Read the model definition and answer for the solid it produces. Units are mm, in the model's axes. Face numbers are marked on the shaded views. A direction names the side the tool comes from. Give positions to 0.01 mm unless a question says otherwise; leave off trailing zeros. Write each loop counter-clockwise with the first axis right and the second up, starting at its lowest first coordinate (ties: lowest second). Pieces come first, ordered by that corner, then holes. Notation, with made-up numbers: (11, -7.5) -> (52, -7.5) arc R18 cw to (52, -3.5) -> close; hole circle Ø3 at (-23, 35). An arc over 180 degrees is marked (long way). Answer as CSV lines item,"result". Start each with the question number.
1. The part is cut by section A-A, the plane z = -3.25. Determine the outline of the cut face in (x, y), and give its area (3 significant figures).
2. The part is cut by section D-D, the plane z = 0. Determine the outline of the cut face in (x, y), and give its area (3 significant figures).
3. The part is cut by section C-C, the plane y = 1.5. Determine the outline of the cut face in (x, z).
4. Find the intervals of material crossed by line 1 (Z direction, x = 0, y = 5); line 2 (Z direction, x = 13, y = -42.5); line 3 (Y direction, x = -19, z = -1.5), in increasing order.
5. A tool of negligible diameter and unlimited length cuts with its end or side. For the marked faces 1, 2, 3, 4 and 5, from which of +Z, -Z, +X, -X, +Y, -Y can it reach the whole face along a straight path? Write none if from no direction.
6. The part is cut by section B-B, the plane x = 0. Determine the outline of the cut face in (y, z), and give its area (3 significant figures).
7. Given pin 1 (1 mm diameter, centred on y = -4, z = 3, fed in from -X); pin 2 (4 mm diameter, centred on x = -6.5, z = 2, fed in from +Y); pin 3 (3 mm diameter, centred on y = -22.5, z = 3.5, fed in from +X), each flat-ended and moving along its own axis, determine where each tip first touches the part or whether it passes through.
8. For a pull along X with two mould halves and no side action, classify the marked faces 6, 7 and 8 as pulls with the +X half, pulls with the -X half, needs draft (parallel to the pull), parting line crosses it, or undercut.
from build123d import *

# Parameters (mm, degrees)
PAD_DEPTH            = 4.5
SKETCH001_R          = 1
POCKET_DEPTH         = 11.302669
POCKET001_DEPTH      = 38.049191
POCKET001_DEPTH_BACK = -38.049191
FILLET_R             = 10


with BuildPart() as part:
    # Sketch → Pad (new body, symmetric)
    with BuildSketch(Plane.XY):
        with BuildLine():
            Line((10, 5.265712), (38.048191, -48))
            Line((-38.048191, -48), (38.048191, -48))
            Line((-38.048191, -48), (-10, 5.265712))
            ThreePointArc((10, 5.265712), (0, 11.301669), (-10, 5.265712))
        make_face()
        with BuildLine():
            Line((-4.76, 0.428554), (-21.895934, -32.113926))
            ThreePointArc((-21.895934, -32.113926), (-21.741576, -37.400351), (-17.135934, -40))
            Line((-17.135934, -40), (17.135934, -40))
            ThreePointArc((17.135934, -40), (21.741576, -37.400351), (21.895934, -32.113926))
            Line((21.895934, -32.113926), (4.76, 0.428554))
            ThreePointArc((4.76, 0.428554), (0, 3.301669), (-4.76, 0.428554))
        make_face(mode=Mode.SUBTRACT)
    extrude(amount=PAD_DEPTH, both=True)

    # Sketch001 → Pocket (cut, through all)
    with BuildSketch(Plane.XZ):
        Circle(SKETCH001_R)
    extrude(amount=-POCKET_DEPTH, mode=Mode.SUBTRACT)

    # Sketch002 → Pocket001 (cut, two sides)
    with BuildSketch(Plane.YZ) as pocket001_sk:
        Polygon((-41, -5.5), (-41, -2.5), (-46, -2.5), (-46, 2.5), (-36, 2.5), (-36, -5.5), align=None)
    extrude(amount=-POCKET001_DEPTH, mode=Mode.SUBTRACT)
    extrude(pocket001_sk.sketch, amount=-POCKET001_DEPTH_BACK, mode=Mode.SUBTRACT)

    # Fillet
    fillet_edges = [part.edges().sort_by_distance(p)[0] for p in [
        (38.048191, -48, 0),
        (-38.048191, -48, 0),
    ]]
    fillet(fillet_edges, radius=FILLET_R)


solid = part.part
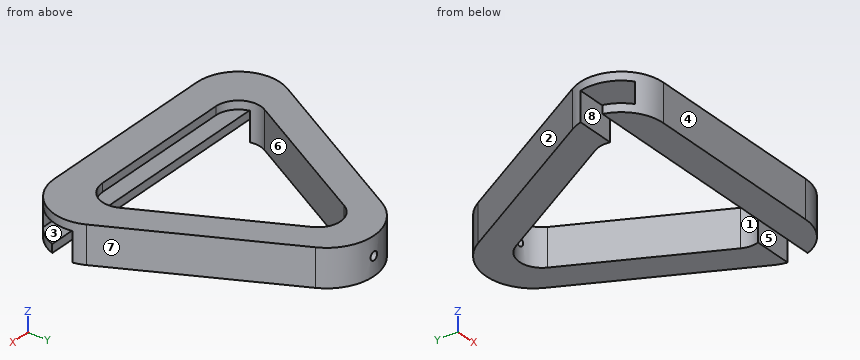
Results found:
1,outline,"(-31.28, -36) -> (-22.34, -36) arc R5.38 cw to (-21.9, -32.11) -> (-4.76, 0.43) arc R5.38 cw to (4.76, 0.43) -> (21.9, -32.11) arc R5.38 cw to (22.34, -36) -> (31.28, -36) arc R10 ccw to (30.33, -33.34) -> (10, 5.27) arc R11.3 ccw to (-10, 5.27) -> (-30.33, -33.34) arc R10 ccw to start; (-31.02, -41) arc R10 ccw to (-21.48, -48) -> (21.48, -48) arc R10 ccw to (31.02, -41) -> close"
1,area,"1,150 mm²"
2,outline,"(-31.28, -36) -> (-22.34, -36) arc R5.38 cw to (-21.9, -32.11) -> (-4.76, 0.43) arc R5.38 cw to (-1, 3.21) -> (-1, 11.26) arc R11.3 ccw to (-10, 5.27) -> (-30.33, -33.34) arc R10 ccw to start; (-27.48, -46) arc R10 ccw to (-21.48, -48) -> (21.48, -48) arc R10 ccw to (27.48, -46) -> close; (1, 3.21) arc R5.38 cw to (4.76, 0.43) -> (21.9, -32.11) arc R5.38 cw to (22.34, -36) -> (31.28, -36) arc R10 ccw to (30.33, -33.34) -> (10, 5.27) arc R11.3 ccw to (1, 11.26) -> close"
2,area,"833 mm²"
3,outline,"(-11.98, -4.5) -> (-4.02, -4.5) -> (-4.02, 4.5) -> (-11.98, 4.5) -> close; (4.02, -4.5) -> (11.98, -4.5) -> (11.98, 4.5) -> (4.02, 4.5) -> close"
4,line 1,"z = -4.5 to -1, 1 to 4.5"
4,line 2,"z = -4.5 to -2.5, 2.5 to 4.5"
4,line 3,"y = -48 to -46, -26.61 to -11.83"
5,face 1,"+Z, -Z"
5,face 2,"+Z, -Z, -X, +Y"
5,face 3,"+X, -X"
5,face 4,"+Z, -Z, +X, -X, -Y"
5,face 5,"-Z, +X, -X"
6,outline,"(-48, -4.5) -> (-41, -4.5) -> (-41, -2.5) -> (-46, -2.5) -> (-46, 2.5) -> (-40, 2.5) -> (-40, 4.5) -> (-48, 4.5) -> close; (3.3, -4.5) -> (11.3, -4.5) -> (11.3, -1) -> (3.3, -1) -> close; (3.3, 1) -> (11.3, 1) -> (11.3, 4.5) -> (3.3, 4.5) -> close"
6,area,"96.0 mm²"
7,pin 1,"stops at x = -15.14"
7,pin 2,"stops at y = 10.37"
7,pin 3,"stops at x = 25.41"
8,face 6,"undercut"
8,face 7,"pulls with the +X half"
8,face 8,"needs draft"
